Design review of the part built by this model. Coordinates are the model's own, in mm. A direction names the side the tool comes from. Round coordinates to 2 decimals unless told otherwise and drop trailing zeros. Loops run counter-clockwise (first coordinate to the right, second up) from the corner with the lowest first, then second, coordinate; pieces in that order, holes last. Notation, with made-up numbers: (9, 46) -> (51, 46) arc R20 ccw to (51, 75) -> close; hole circle Ø1 at (40, 12.5). An arc over 180 degrees is marked (long way). Use a Markdown table: item, result. Add a question column.
from build123d import *

# Parameters (mm, degrees)
BOX003_W                    = 4
BOX003_H                    = 4
BOX003_DEPTH                = 5
BOX003_PITCH_ANGLE          = 90
BOX003_PLACEMENT_ANGLE      = 17.5
BOX004_W                    = 4
BOX004_H                    = 4
BOX004_DEPTH                = 5
BOX004_PITCH_ANGLE          = 90
BOX004_PLACEMENT_ANGLE      = -17.5
BOX005_W                    = 4
BOX005_H                    = 4
BOX005_DEPTH                = 5
BOX005_PITCH_ANGLE          = 90
BOX005_PLACEMENT_ANGLE      = -52.5
BOX006_W                    = 4
BOX006_H                    = 4
BOX006_DEPTH                = 5
BOX006_PITCH_ANGLE          = 90
BOX006_PLACEMENT_ANGLE      = 52.5
CYLINDER004_R               = 2.8
CYLINDER004_DEPTH           = 10
CYLINDER004_PITCH_ANGLE     = 90
CYLINDER004_PLACEMENT_ANGLE = 17.5
CYLINDER005_R               = 2.8
CYLINDER005_DEPTH           = 10
CYLINDER005_PITCH_ANGLE     = 90
CYLINDER005_PLACEMENT_ANGLE = -17.5
CYLINDER006_R               = 2.8
CYLINDER006_DEPTH           = 10
CYLINDER006_PITCH_ANGLE     = 90
CYLINDER006_PLACEMENT_ANGLE = -52.5
CYLINDER007_R               = 2.8
CYLINDER007_DEPTH           = 10
CYLINDER007_PITCH_ANGLE     = 90
CYLINDER007_PLACEMENT_ANGLE = 52.5
SKETCH010_R                 = 20
PAD004_DEPTH                = 4
PAD005_DEPTH                = 8
SKETCH012_R                 = 4
POCKET006_DEPTH             = 2
SKETCH013_R                 = 2.4
POCKET007_DEPTH             = 2
SKETCH050_R                 = 4
POCKET023_DEPTH             = 5


with BuildPart() as box003:
    # Box003 → Box003 (new body)
    with BuildSketch(Plane.XY):
        with Locations((2, 2)):
            Rectangle(BOX003_W, BOX003_H)
    extrude(amount=BOX003_DEPTH)


with BuildPart() as box003_1:
    # Box003 pitch: moved
    add(box003.part.rotate(Axis((0, 0, 0), (0, 1, 0)), BOX003_PITCH_ANGLE))


with BuildPart() as box003_2:
    # Box003 placement: moved
    add(box003_1.part.moved(Location((16.5733556333, -8.2222556911, 18.5))).rotate(Axis((16.5733556333, -8.2222556911, 18.5), (0, 0, 1)), BOX003_PLACEMENT_ANGLE))


with BuildPart() as box004:
    # Box004 → Box004 (new body)
    with BuildSketch(Plane.XY):
        with Locations((2, 2)):
            Rectangle(BOX004_W, BOX004_H)
    extrude(amount=BOX004_DEPTH)


with BuildPart() as box004_1:
    # Box004 pitch: moved
    add(box004.part.rotate(Axis((0, 0, 0), (0, 1, 0)), BOX004_PITCH_ANGLE))


with BuildPart() as box004_2:
    # Box004 placement: moved
    add(box004_1.part.moved(Location((15.3705324353, 4.4073878881, 18.5))).rotate(Axis((15.3705324353, 4.4073878881, 18.5), (0, 0, 1)), BOX004_PLACEMENT_ANGLE))


with BuildPart() as box005:
    # Box005 → Box005 (new body)
    with BuildSketch(Plane.XY):
        with Locations((2, 2)):
            Rectangle(BOX005_W, BOX005_H)
    extrude(amount=BOX005_DEPTH)


with BuildPart() as box005_1:
    # Box005 pitch: moved
    add(box005.part.rotate(Axis((0, 0, 0), (0, 1, 0)), BOX005_PITCH_ANGLE))


with BuildPart() as box005_2:
    # Box005 placement: moved
    add(box005_1.part.moved(Location((21.6293033102, 15.4428972881, 18.5))).rotate(Axis((21.6293033102, 15.4428972881, 18.5), (0, 0, 1)), BOX005_PLACEMENT_ANGLE))


with BuildPart() as fusion:
    # Box006 → Box006 (new body)
    with BuildSketch(Plane.XY):
        with Locations((2, 2)):
            Rectangle(BOX006_W, BOX006_H)
    extrude(amount=BOX006_DEPTH)


with BuildPart() as fusion_1:
    # Box006 pitch: moved
    add(fusion.part.rotate(Axis((0, 0, 0), (0, 1, 0)), BOX006_PITCH_ANGLE))


with BuildPart() as fusion_2:
    # Box006 placement: moved
    add(fusion_1.part.moved(Location((24.8027166714, -17.8779430041, 18.5))).rotate(Axis((24.8027166714, -17.8779430041, 18.5), (0, 0, 1)), BOX006_PLACEMENT_ANGLE))

    # Fusion: union Box003, Box004, Box005
    add(box003_2.part)
    add(box004_2.part)
    add(box005_2.part)


with BuildPart() as cylinder004:
    # Cylinder004 → Cylinder004 (new body)
    with BuildSketch(Plane.XY):
        Circle(CYLINDER004_R)
    extrude(amount=CYLINDER004_DEPTH)


with BuildPart() as cylinder004_1:
    # Cylinder004 pitch: moved
    add(cylinder004.part.rotate(Axis((0, 0, 0), (0, 1, 0)), CYLINDER004_PITCH_ANGLE))


with BuildPart() as cylinder004_2:
    # Cylinder004 placement: moved
    add(cylinder004_1.part.moved(Location((15.9719440343, -6.3148217896, 26))).rotate(Axis((15.9719440343, -6.3148217896, 26), (0, 0, 1)), CYLINDER004_PLACEMENT_ANGLE))


with BuildPart() as cylinder005:
    # Cylinder005 → Cylinder005 (new body)
    with BuildSketch(Plane.XY):
        Circle(CYLINDER005_R)
    extrude(amount=CYLINDER005_DEPTH)


with BuildPart() as cylinder005_1:
    # Cylinder005 pitch: moved
    add(cylinder005.part.rotate(Axis((0, 0, 0), (0, 1, 0)), CYLINDER005_PITCH_ANGLE))


with BuildPart() as cylinder005_2:
    # Cylinder005 placement: moved
    add(cylinder005_1.part.moved(Location((15.9719440343, 6.3148217896, 26))).rotate(Axis((15.9719440343, 6.3148217896, 26), (0, 0, 1)), CYLINDER005_PLACEMENT_ANGLE))


with BuildPart() as cylinder006:
    # Cylinder006 → Cylinder006 (new body)
    with BuildSketch(Plane.XY):
        Circle(CYLINDER006_R)
    extrude(amount=CYLINDER006_DEPTH)


with BuildPart() as cylinder006_1:
    # Cylinder006 pitch: moved
    add(cylinder006.part.rotate(Axis((0, 0, 0), (0, 1, 0)), CYLINDER006_PITCH_ANGLE))


with BuildPart() as cylinder006_2:
    # Cylinder006 placement: moved
    add(cylinder006_1.part.moved(Location((23.2160099908, 16.6604201461, 26))).rotate(Axis((23.2160099908, 16.6604201461, 26), (0, 0, 1)), CYLINDER006_PLACEMENT_ANGLE))


with BuildPart() as fusion002:
    # Cylinder007 → Cylinder007 (new body)
    with BuildSketch(Plane.XY):
        Circle(CYLINDER007_R)
    extrude(amount=CYLINDER007_DEPTH)


with BuildPart() as fusion002_1:
    # Cylinder007 pitch: moved
    add(fusion002.part.rotate(Axis((0, 0, 0), (0, 1, 0)), CYLINDER007_PITCH_ANGLE))


with BuildPart() as fusion002_2:
    # Cylinder007 placement: moved
    add(fusion002_1.part.moved(Location((23.2160099908, -16.6604201461, 26))).rotate(Axis((23.2160099908, -16.6604201461, 26), (0, 0, 1)), CYLINDER007_PLACEMENT_ANGLE))

    # Fusion001: union Cylinder004, Cylinder005, Cylinder006
    add(cylinder004_2.part)
    add(cylinder005_2.part)
    add(cylinder006_2.part)


with BuildPart() as cut001:
    # Sketch010 (on Face1 of CopyPocket005) → Pad004 (new body)
    with BuildSketch(Plane.XY.offset(18)):
        with Locations((36, 0)):
            Circle(SKETCH010_R)
    extrude(amount=PAD004_DEPTH)

    # Sketch011 (on Face3 of Pad004) → Pad005 (join)
    with BuildSketch(Plane.XY.offset(22)):
        with BuildLine():
            ThreePointArc((29.1595971335, 18.7938524157), (16, 0), (29.1595971335, -18.7938524157))
            Line((31.2117179934, -13.155696691), (29.1595971335, -18.7938524157))
            ThreePointArc((31.2117179934, 13.155696691), (22, 0), (31.2117179934, -13.155696691))
            Line((31.2117179934, 13.155696691), (29.1595971335, 18.7938524157))
        make_face()
    extrude(amount=PAD005_DEPTH)

    # Sketch012 (on Face3 of Pad005) → Pocket006 (cut)
    with BuildSketch(Plane.XY.offset(22)):
        with Locations((36, 0)):
            Circle(SKETCH012_R)
    extrude(amount=-POCKET006_DEPTH, mode=Mode.SUBTRACT)

    # Sketch013 (on Face10 of Pocket006) → Pocket007 (cut)
    with BuildSketch(Plane.XY.offset(20)):
        with Locations((36, 0)):
            Circle(SKETCH013_R)
    extrude(amount=-POCKET007_DEPTH, mode=Mode.SUBTRACT)

    # Sketch050 (on Face4 of Pocket007) → Pocket023 (cut)
    with BuildSketch(Plane.XY.offset(22)):
        with Locations((43.5244431532, 20.6732376573)):
            Circle(SKETCH050_R)
        with Locations((54.0213449744, 12.6186815997)):
            Circle(SKETCH050_R)
        with Locations((58, 0)):
            Circle(SKETCH050_R)
        with Locations((54.0213449744, -12.6186815997)):
            Circle(SKETCH050_R)
        with Locations((43.5244431532, -20.6732376573)):
            Circle(SKETCH050_R)
    extrude(amount=-POCKET023_DEPTH, mode=Mode.SUBTRACT)

    # Cut: cut Fusion002
    add(fusion002_2.part, mode=Mode.SUBTRACT)

    # Cut001: cut Fusion
    add(fusion_2.part, mode=Mode.SUBTRACT)


solid = cut001.part
1. Consider section D-D on z = 25.5. State the section outline as (x, y) points.
2. Consider section C-C on y = 0. State the section outline as (x, z) points.
3. Insertion check: P1, Ø3, axis at y = -2, z = 20, coming from the -X side; P2, Ø6, axis at x = 25.5, y = -14, coming from the -Z side; P3, Ø10.5, axis at x = 36, y = 0, coming from the +Z side; P4, Ø6, axis at x = 39.5, z = 20.5, coming from the -Y side. Each pin has a flat end and moves straight along its axis. Give the tip position at first contact, or say it passes through.
4. Consider section A-A on x = 36. State the section outline as (y, z) points.
5. Consider section B-B on z = 20.5. State the section outline as (x, y) points, plus the area to 3 significant figures.
6. For faces 5 (the face through (42, 0, 22)), 6 (the face through (23.469, -13.045, 18.254)), 7 (the face through (26.24, -12.68, 18.25)), 8 (the face through (19.5, -7.3, 18.3)), 9 (the face through (19.8, -5, 28.8)), list the 3-axis set-ups (+Z, -Z, +X, -X, +Y, -Y) from which the entire face can be reached by the end or side of a thin tool; tool diameter is ignored.
7. Mouldability with a two-part tool opening along Y and no side actions: class faces 1 (the face through (21.8, 0.3, 30)), 2 (the face through (25.612, -13.336, 28.797)), 3 (the face through (42.2, -16.9, 20)), 4 (the face through (48, 16, 20)) as +Y half, -Y half, draft (parallel to the pull), parting line (faces both ways), or undercut.
8. To check wall thickness, follow probe 1 along Y at (x, z) = (36, 19); probe 2 along Z at (x, y) = (40, -12); probe 3 along X at (y, z) = (2, 20.5). State the ranges of each line that lie inside material, in increasing order. Write a range as from..to.
Verdict:
| question | item | result |
|---|---|---|
| 1 | outline | (16.28, -3.33) -> (22.08, -1.5) arc R14 cw to (22.08, 1.5) -> (16.28, 3.33) arc R20 ccw to start; (17.94, -8.58) arc R20 ccw to (21.76, -14.04) -> (25.46, -9.21) arc R14 cw to (23.74, -6.76) -> close; (17.94, 8.58) -> (23.74, 6.76) arc R14 cw to (25.46, 9.21) -> (21.76, 14.04) arc R20 ccw to start; (26.13, -17.39) arc R20 ccw to (29.16, -18.79) -> (31.21, -13.16) arc R14 cw to (29.83, -12.57) -> close; (26.13, 17.39) -> (29.83, 12.57) arc R14 cw to (31.21, 13.16) -> (29.16, 18.79) arc R20 ccw to start |
| 2 | outline | (16, 18) -> (33.6, 18) -> (33.6, 20) -> (32, 20) -> (32, 22) -> (22, 22) -> (22, 30) -> (16, 30) -> close; (38.4, 18) -> (54, 18) -> (54, 22) -> (40, 22) -> (40, 20) -> (38.4, 20) -> close |
| 3 | P1 | stops at x = 16.01 |
| 3 | P2 | stops at z = 18 |
| 3 | P3 | stops at z = 22 |
| 3 | P4 | stops at y = -19.99 |
| 4 | outline | (-20, 18) -> (-2.4, 18) -> (-2.4, 20) -> (-4, 20) -> (-4, 22) -> (-20, 22) -> close; (2.4, 18) -> (20, 18) -> (20, 22) -> (4, 22) -> (4, 20) -> (2.4, 20) -> close |
| 5 | outline | (39.65, -19.66) arc R4 cw to (45.84, -17.41) arc R20 ccw to (50.27, -14.01) arc R4 cw to (54.05, -8.62) arc R20 ccw to (55.73, -3.29) arc R4 cw to (55.73, 3.29) arc R20 ccw to (54.05, 8.62) arc R4 cw to (50.27, 14.01) arc R20 ccw to (45.84, 17.41) arc R4 cw to (39.65, 19.66) arc R20 ccw (long way) to start; hole circle Ø8 at (36, 0) |
| 5 | area | 1,160 mm² |
| 6 | face 5 | +Z, +X |
| 6 | face 6 | -Z, -Y |
| 6 | face 7 | -Z |
| 6 | face 8 | -Z, -X |
| 6 | face 9 | none |
| 7 | face 1 | draft |
| 7 | face 2 | undercut |
| 7 | face 3 | -Y half |
| 7 | face 4 | +Y half |
| 8 | probe 1 | y = -20..-2.4, 2.4..20 |
| 8 | probe 2 | z = 18..22 |
| 8 | probe 3 | x = 16.1..32.54, 39.46..54.54 |
